The model under review builds one solid part; all positions refer to its coordinate system, in mm. Coordinates: 2 decimals unless noted, no trailing zeros. Loops run counter-clockwise (first coordinate to the right, second up) from the corner with the lowest first, then second, coordinate; pieces in that order, holes last. Notation, with made-up numbers: M 18.5,5.25 L 27.5,5.25 A21 ccw 27.5,12.25 Z; hole C 73,89.25 d1. An arc over 180 degrees is marked long. Return JSON: item names as keys, results as strings.
```python
from build123d import *

# Parameters (mm, degrees)
MODEL_R                           = 3.999999997
BOSS_EXTRUDE1_DEPTH               = 381
F_3_8_16_TAPPED_HOLE1_D           = 7.9375
F_3_8_16_TAPPED_HOLE1_CSINK_D     = 10.16
F_3_8_16_TAPPED_HOLE1_CSINK_ANGLE = 90


with BuildPart() as part:
    # Model → Boss-Extrude1 (new body)
    with BuildSketch(Plane.XY):
        with BuildLine():
            Line((-18.843780991, 7.981867858), (-20.966888929, 12.534890876))
            ThreePointArc((-20.966888929, 12.534890876), (-21.047789267, 12.798072701), (-21.053849819, 13.07334131))
            ThreePointArc((-21.053849819, 13.07334131), (-34.474612004, 19.833405747), (-28.578947374, 6.011088019))
            ThreePointArc((-28.578947374, 6.011088019), (-27.4676292, 5.601381399), (-27.000000001, 4.513167022))
            Line((-27.000000001, 4.513167022), (-27.000000001, 0.700000022))
            Line((-27.000000001, 0.700000022), (-26.500000001, 0.200000022))
            Line((-26.500000001, 0.200000022), (-20.200001001, 0.200000022))
            Line((-20.200001001, 0.200000022), (-20.000000979, 0))
            Line((-20.000000979, 0), (-6.000000502, 0))
            Line((-6.000000502, 0), (-5.80000048, 0.200000022))
            Line((-5.80000048, 0.200000022), (5.80000048, 0.200000022))
            Line((5.80000048, 0.200000022), (6.000000502, 0))
            Line((6.000000502, 0), (20.000000979, 0))
            Line((20.000000979, 0), (20.200001001, 0.200000022))
            Line((20.200001001, 0.200000022), (26.500000001, 0.200000022))
            Line((26.500000001, 0.200000022), (27.000000001, 0.700000022))
            Line((27.000000001, 0.700000022), (27.000000001, 4.513167022))
            ThreePointArc((27.000000001, 4.513167022), (27.4676292, 5.601381399), (28.578947374, 6.011088019))
            ThreePointArc((28.578947374, 6.011088019), (34.474612004, 19.833405747), (21.053849819, 13.07334131))
            ThreePointArc((21.053849819, 13.07334131), (21.047789267, 12.798072701), (20.966888929, 12.534890876))
            Line((20.966888929, 12.534890876), (18.843780991, 7.981867858))
            ThreePointArc((18.843780991, 7.981867858), (18.479330527, 7.628755749), (17.98848008, 7.499999621))
            Line((17.98848008, 7.499999621), (0.500000254, 7.499999621))
            Line((0.500000254, 7.499999621), (0, 7.211324621))
            Line((0, 7.211324621), (-0.500000254, 7.499999621))
            Line((-0.500000254, 7.499999621), (-17.98848008, 7.499999621))
            ThreePointArc((-17.98848008, 7.499999621), (-18.479330527, 7.628755749), (-18.843780991, 7.981867858))
        make_face()
        with Locations((-29.000000026, 13.999999962)):
            Circle(MODEL_R, mode=Mode.SUBTRACT)
        with Locations((29.000000026, 13.999999962)):
            Circle(MODEL_R, mode=Mode.SUBTRACT)
    extrude(amount=BOSS_EXTRUDE1_DEPTH)

    # 3/8-16 Tapped Hole1 (through all)
    with Locations(Plane(origin=(0, 7.499999621, 0), x_dir=(1, 0, 0), z_dir=(0, 1, 0))):
        with Locations((0, -25.4), (0, -127), (0, -228.6), (0, -330.2), (0, -431.8), (0, -533.4), (0, -635), (0, -736.6), (0, -838.2), (0, -939.8), (0, -1041.4), (0, -1143), (0, -1244.6), (0, -1346.2), (0, -1447.8), (0, -1549.4), (0, -1651), (0, -1752.6), (0, -1854.2), (0, -1955.8)):
            CounterSinkHole(F_3_8_16_TAPPED_HOLE1_D / 2, F_3_8_16_TAPPED_HOLE1_CSINK_D / 2, counter_sink_angle=F_3_8_16_TAPPED_HOLE1_CSINK_ANGLE)


solid = part.part
```
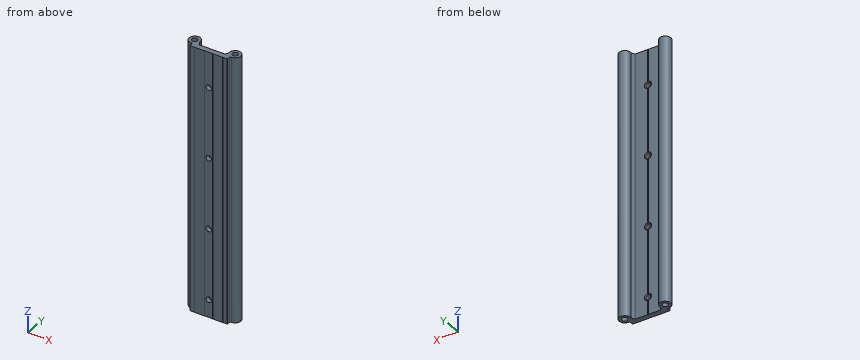
1. Insertion check: pin 1 Ø1.9 at (y, z) = (3, 211.5) entering from +X; pin 2 Ø19 at (x, z) = (10, 216.5) entering from +Y; pin 3 Ø6 at (y, z) = (8, 57.5) entering from +X; pin 4 Ø6.5 at (x, z) = (0, 330.2) entering from +Y. Each pin has a flat end and moves straight along its axis. Give the tip position at first contact, or say it passes through.
Check values:
{"pin 1": "x = 27", "pin 2": "y = 9.39", "pin 3": "x = 36.42", "pin 4": "through"}
2. To check wall thickness, follow line 1 (X direction, y = 14, z = 304.5); line 2 (Z direction, x = 0, y = 3.75); line 3 (Y direction, x = 29, z = 112). State the ranges of each line that lie inside material, in increasing order.
Check values:
{"line 1": "-37 to -33, -25 to -21, 21 to 25, 33 to 37", "line 2": "0 to 21.43, 29.37 to 123.03, 130.97 to 224.63, 232.57 to 326.23, 334.17 to 381", "line 3": "6 to 10, 18 to 22"}
3. Add section C-C on x = -10. Give the boundary of the cut face in (y, z), plus the area to 3 significant figures.
Check values:
{"outline": "M 0,0 L 7.5,0 L 7.5,381 L 0,381 Z", "area": "2,860 mm²"}
4. Add section A-A on z = 25.4. State how many separate pieces and enclosed holes the cut face has, plus the area to 3 significant figures.
Check values:
{"separate pieces": "2", "enclosed holes": "2", "area": "665 mm²"}
